Autodesk Inventor part; units mm, degrees
ref_plane "YZ Plane" through (0, 0, 0) normal (1, 0, 0) x (0, 1, 0)
ref_plane "XZ Plane" through (0, 0, 0) normal (0, 1, 0) x (-1, 0, 0)
ref_plane "XY Plane" through (0, 0, 0) normal (0, 0, 1) x (1, 0, 0)
sketch "Sketch1" plane through (0, 0, 0) normal (0, 0, 1) x (1, 0, 0)
  line L0 (0, 0) -> (39, 0)
  line L1 (0, 0) -> (0, 10)
  line L2 (39, 0) -> (39, 10)
  line L3 (0, 10) -> (9.5, 19.5)
  line L4 (39, 10) -> (29.5, 19.5)
  line L5 (9.5, 24.2513) -> (2, 31.7513)
  line L6 (2, 31.7513) -> (2, 46.2487)
  line L7 (2, 46.2487) -> (12.2513, 56.5)
  line L8 (12.2513, 56.5) -> (26.7487, 56.5)
  line L9 (26.7487, 56.5) -> (37, 46.2487)
  line L10 (37, 46.2487) -> (37, 31.7513)
  line L11 (37, 31.7513) -> (29.5, 24.2513)
  line L12 (23.6421, 29) -> (15.3579, 29)
  line L13 (15.3579, 29) -> (9.5, 34.8579)
  line L14 (9.5, 34.8579) -> (9.5, 43.1421)
  line L15 (9.5, 43.1421) -> (15.3579, 49)
  line L16 (15.3579, 49) -> (23.6421, 49)
  line L17 (23.6421, 49) -> (29.5, 43.1421)
  line L18 (29.5, 43.1421) -> (29.5, 34.8579)
  line L19 (29.5, 34.8579) -> (23.6421, 29)
  line L20 (9.5, 19.5) -> (9.5, 24.2513)
  line L21 (29.5, 19.5) -> (29.5, 24.2513)
  point P0 (19.5, 39)
  point P1 (19.5, 39)
  point P2 (19.5, 0)
  dimension "d0" = 39
  dimension "d1" = 45
  dimension "d2" = 39
  dimension "d3" = 20
  dimension "d4" = 35
  dimension "d5" = 10
  dimension "d6" = 20
extrude "Extrusion1" add sketch "Sketch1" along normal blind 6
sketch "Sketch2" plane through (0, 0, 6) normal (0, 0, 1) x (1, 0, 0)
  line L0 (0, 0) -> (39, 0)
  line L1 (17.25, 16.3) -> (21.75, 16.3)
  line L2 (21.75, 0) -> (17.25, 0)
  line L3 (24.25, 12.3) -> (24.25, 5)
  line L4 (14.75, 5) -> (14.75, 12.3)
  line L5 (21.75, 16.3) -> (21.75, 12.3)
  line L6 (21.75, 5) -> (21.75, 0)
  line L7 (17.25, 0) -> (17.25, 5)
  line L8 (17.25, 12.3) -> (17.25, 16.3)
  line L9 (14.75, 12.3) -> (17.25, 12.3)
  line L10 (21.75, 12.3) -> (24.25, 12.3)
  line L11 (24.25, 5) -> (21.75, 5)
  line L12 (17.25, 5) -> (14.75, 5)
  point P0 (19.5, 16.3)
  point P1 (19.5, 0)
  dimension "d9" = 5
  dimension "d10" = 4
  dimension "d11" = 7.3
  dimension "d12" = 2.5
  dimension "d13" = 2.5
  dimension "d14" = 4.5
extrude "Extrusion2" cut sketch "Sketch2" against normal blind 6
sketch "Sketch3" plane through (0, 0, 6) normal (0, 0, 1) x (1, 0, 0)
  line L0 (21.75, 0) -> (39, 0)
  line L1 (0, 0) -> (17.25, 0)
  line L2 (17.25, 16.3) -> (21.75, 16.3)
  line L3 (4, 0) -> (12, 0)
  line L4 (12, 0) -> (12, -4)
  line L5 (10, -6) -> (6, -6)
  line L6 (4, -4) -> (4, 0)
  line L7 (27, 0) -> (35, 0)
  line L8 (35, 0) -> (35, -4)
  line L9 (33, -6) -> (29, -6)
  line L10 (27, -4) -> (27, 0)
  arc A0 (4, -4) -> (6, -6) centre (6, -4) ccw
  arc A1 (10, -6) -> (12, -4) centre (10, -4) ccw
  arc A2 (27, -4) -> (29, -6) centre (29, -4) ccw
  arc A3 (33, -6) -> (35, -4) centre (33, -4) ccw
  point P0 (19.5, 16.3)
  dimension "d17" = 2
  dimension "d18" = 8
  dimension "d19" = 8
  dimension "d20" = 6
  dimension "d21" = 7.5
  dimension "d22" = 15
extrude "Extrusion3" add sketch "Sketch3" against normal blind 6
properties part number "filament_guide"
Model file for the job. Use its own axes, mm. A direction names the side the tool comes from. Give positions to 0.01 mm unless a question says otherwise; leave off trailing zeros. Loops run counter-clockwise (first coordinate to the right, second up) from the corner with the lowest first, then second, coordinate; pieces in that order, holes last.
1) Saw through at A-A (y = 9). Write the cut outline in (x, z), plus the area to 3 significant figures.
2) Flat gauge pins, fed straight in: pin 1 Ø1.8 at (y, z) = (38, 4.5) entering from +X; pin 2 Ø1 at (y, z) = (47.5, 4.5) entering from -X; pin 3 Ø1.2 at (y, z) = (-1, 3.5) entering from -X. Where does each tip first touch, or does it go through?
3) Saw through at C-C (y = 22). Write the cut outline in (x, z).
4) Saw through at B-B (x = 21). Write the cut outline in (y, z), plus the area to 3 significant figures.
5) Wall check: line 1 (X direction, y = 3, z = 1.2); line 2 (X direction, y = 7, z = 5.2); line 3 (Y direction, x = 15, z = 4.85). Give the ranges that are in metal, low to high.
6) Pull direction Y, two halves, no side cores. Call faces 1 (the flat face through (5, 15, 3)), 2 (the flat face through (12, -2, 3)), 3 (the flat face through (15, 0, 3)): +Y half, -Y half, draft (parallel to the pull), parting line (faces both ways), or undercut.
7) Tool access for faces 4 (the flat face through (37, 0, 3)), 5 (the flat face through (14.75, 9, 3)), 6 (the flat face through (2, 0, 3)), 7 (the flat face through (37, 39, 3)), 8 (the flat face through (29.5, 22, 3)): list every direction of +Z, -Z, +X, -X, +Y, -Y with a clear straight run to the whole face (end or side of a thin tool).
Answer block:
1. outline: (0, 0) - (14.75, 0) - (14.75, 6) - (0, 6) - close; (24.25, 0) - (39, 0) - (39, 6) - (24.25, 6) - close
1. area: 177 mm2
2. pin 1: stops at x = 37
2. pin 2: stops at x = 2.75
2. pin 3: stops at x = 4
3. outline: (9.5, 0) - (29.5, 0) - (29.5, 6) - (9.5, 6) - close
4. outline: (16.3, 0) - (29, 0) - (29, 6) - (16.3, 6) - close; (49, 0) - (56.5, 0) - (56.5, 6) - (49, 6) - close
4. area: 121 mm2
5. line 1: x = 0 to 17.25, 21.75 to 39
5. line 2: x = 0 to 14.75, 24.25 to 39
5. line 3: y = 0 to 5, 12.3 to 29.36, 48.64 to 56.5
6. face 1: undercut
6. face 2: draft
6. face 3: -Y half
7. face 4: +Z, -Z, +X, -Y
7. face 5: +Z, -Z
7. face 6: +Z, -Z, -X, -Y
7. face 7: +Z, -Z, +X, +Y
7. face 8: +Z, -Z, +X
